```python
from build123d import *

# Parameters (mm, degrees)
BOSS_EXTRUDE1_DEPTH = 6.35
CUT_EXTRUDE1_REACH  = 29.861
SKETCH2_R           = 2.286
CUT_EXTRUDE2_REACH  = 29.861
SKETCH3_R           = 1.905
FILLET1_R           = 4.7625
FILLET2_R           = 6.35
FILLET3_R           = 0.79375


with BuildPart() as part:
    # Sketch1 → Boss-Extrude1 (new body)
    with BuildSketch(Plane(origin=(0, 0, 0), x_dir=(0, 0, -1), z_dir=(1, 0, 0))):
        with BuildLine():
            Line((0, -25.4), (0, 25.4))
            Line((0, 25.4), (-9.525, 25.4))
            Line((-9.525, 25.4), (-9.525, 12.7))
            ThreePointArc((-9.525, 12.7), (-6.35, 0), (-9.525, -12.7))
            Line((-9.525, -12.7), (-9.525, -25.4))
            Line((-9.525, -25.4), (0, -25.4))
        make_face()
    extrude(amount=BOSS_EXTRUDE1_DEPTH)

    # Sketch2 → Cut-Extrude1 (cut, up to next)
    with BuildSketch(Plane.XY.offset(9.525), mode=Mode.PRIVATE) as cut_extrude1_sk1:
        with Locations((2.38125, 19.05)):
            Circle(SKETCH2_R)
    cut_extrude1_tool1 = extrude(cut_extrude1_sk1.sketch, amount=-CUT_EXTRUDE1_REACH, mode=Mode.PRIVATE) & part.part
    # Sketch2 → Cut-Extrude1 (cut, up to next)
    with BuildSketch(Plane.XY.offset(9.525), mode=Mode.PRIVATE) as cut_extrude1_sk2:
        with Locations((2.38125, -19.05)):
            Circle(SKETCH2_R)
    cut_extrude1_tool2 = extrude(cut_extrude1_sk2.sketch, amount=-CUT_EXTRUDE1_REACH, mode=Mode.PRIVATE) & part.part
    add(cut_extrude1_tool1.solids().sort_by_distance((2.38125, 19.05, 9.525))[0], mode=Mode.SUBTRACT)
    add(cut_extrude1_tool2.solids().sort_by_distance((2.38125, -19.05, 9.525))[0], mode=Mode.SUBTRACT)

    # Sketch3 → Cut-Extrude2 (cut, up to next)
    with BuildSketch(Plane(origin=(6.35, 0, 0), x_dir=(0, 0, -1), z_dir=(1, 0, 0)), mode=Mode.PRIVATE) as cut_extrude2_sk1:
        with Locations((-4.7625, 12.7)):
            Circle(SKETCH3_R)
    cut_extrude2_tool1 = extrude(cut_extrude2_sk1.sketch, amount=-CUT_EXTRUDE2_REACH, mode=Mode.PRIVATE) & part.part
    # Sketch3 → Cut-Extrude2 (cut, up to next)
    with BuildSketch(Plane(origin=(6.35, 0, 0), x_dir=(0, 0, -1), z_dir=(1, 0, 0)), mode=Mode.PRIVATE) as cut_extrude2_sk2:
        with Locations((-4.7625, -12.7)):
            Circle(SKETCH3_R)
    cut_extrude2_tool2 = extrude(cut_extrude2_sk2.sketch, amount=-CUT_EXTRUDE2_REACH, mode=Mode.PRIVATE) & part.part
    add(cut_extrude2_tool1.solids().sort_by_distance((6.35, 12.7, 4.7625))[0], mode=Mode.SUBTRACT)
    add(cut_extrude2_tool2.solids().sort_by_distance((6.35, -12.7, 4.7625))[0], mode=Mode.SUBTRACT)

    # Fillet1
    fillet1_edges = [part.edges().sort_by_distance(p)[0] for p in [
        (6.35, 25.4, 4.7625),
        (6.35, -25.4, 4.7625),
    ]]
    fillet(fillet1_edges, radius=FILLET1_R)

    # Fillet2
    fillet2_edges = [part.edges().sort_by_distance(p)[0] for p in [
        (3.175, -12.7, 9.525),
        (3.175, 12.7, 9.525),
    ]]
    fillet(fillet2_edges, radius=FILLET2_R)

    # Fillet3
    fillet3_edges = [part.edges().sort_by_distance(p)[0] for p in [
        (6.35, 17.418265829, 9.525),
        (0.79375, -25.4, 9.525),
        (4.955096045, -24.005096045, 9.525),
        (0.79375, 25.4, 9.525),
        (4.955096045, 24.005096045, 9.525),
        (6.35, -17.418265829, 9.525),
        (6.35, 0, 6.35),
        (6.35, 12.813348054, 9.371965463),
        (6.35, -12.813348054, 9.371965463),
    ]]
    fillet(fillet3_edges, radius=FILLET3_R)


solid = part.part
```
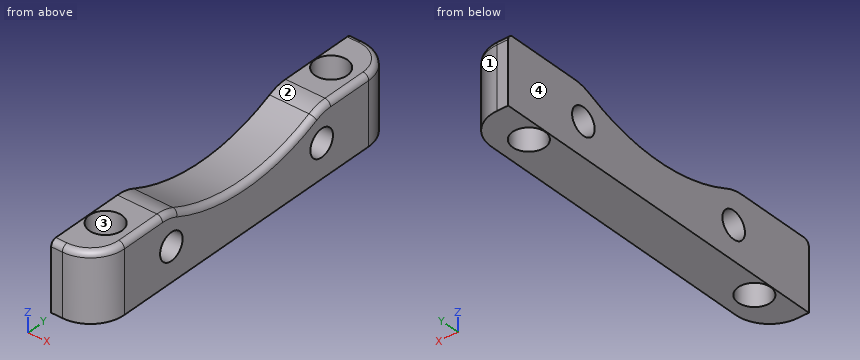
Geometry check sheet. Reference: the model listing, model coordinates, mm. Face numbers are marked on the shaded views. Give positions to 0.01 mm unless a question says otherwise; leave off trailing zeros. Write each question's results on one line, items separated by ' | '. Start each with the question number.
(1) Scan lines: line 1 (Y direction, x = 1.25, z = 0.5); line 2 (Y direction, x = 3.25, z = 4); line 3 (Y direction, x = 1, z = 6). Record each from-to range of solid material in increasing order.
(2) Gauge pin test, flat end, axial feed: P1, Ø3, axis at x = 1.5, y = -5, coming from the +Z side. Record the tip position at first contact, or that the pin passes through.
(3) Mould release check, pull along Y, two halves, no side actions. Record for the marked faces 1, 2, 3 and 4: pulls with the +Y half, pulls with the -Y half, needs draft (parallel to the pull), parting line crosses it, or undercut.
(4) Sectioned sample at A-A (z = 4). Give the number of separate pieces and of enclosed holes in the cut face, plus the area to 3 significant figures.
Answer below:
1) line 1: -25.4 to -21.04, -17.06 to 17.06, 21.04 to 25.4 | line 2: -25.1 to -21.16, -16.94 to -14.45, -10.95 to 10.95, 14.45 to 16.94, 21.16 to 25.1 | line 3: -25.4 to -20.87, -17.23 to -14.15, -11.25 to 11.25, 14.15 to 17.23, 20.87 to 25.4
2) P1: z = 7.14
3) face 1: pulls with the +Y half | face 2: undercut | face 3: undercut | face 4: needs draft
4) separate pieces: 3 | enclosed holes: 2 | area: 236 mm2
